Geometry check sheet. Reference: the model listing, model coordinates, mm. Face numbers are marked on the shaded views. A direction names the side the tool comes from. Coordinates: 2 decimals unless noted, no trailing zeros. Loops run counter-clockwise (first coordinate to the right, second up) from the corner with the lowest first, then second, coordinate; pieces in that order, holes last.
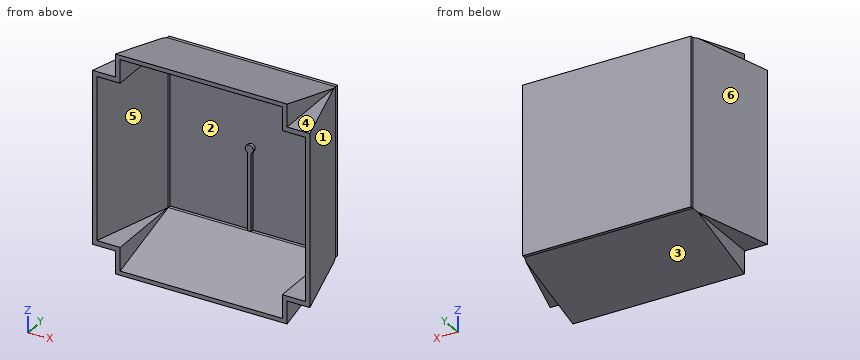
from build123d import *

# Parameters (mm, degrees)
SALIENTE_EXTRUIR1_DEPTH    = 67
CORTAR_EXTRUIR1_DEPTH      = 107
CORTAR_EXTRUIR2_DEPTH      = 107
CORTAR_EXTRUIR3_DEPTH      = 25
CORTAR_EXTRUIR3_DEPTH_BACK = 25
CORTAR_EXTRUIR4_DEPTH      = 25
CORTAR_EXTRUIR4_DEPTH_BACK = 25
CROQUIS14_W                = 7
CROQUIS14_H                = 7
CORTAR_EXTRUIR6_DEPTH      = 70
CROQUIS15_W                = 52
CROQUIS15_H                = 52
SALIENTE_EXTRUIR10_DEPTH   = 1


with BuildPart() as part:
    # Croquis1 → Saliente-Extruir1 (new body)
    with BuildSketch(Plane.XY):
        Polygon((0, 0), (67, 0), (59.5, 26), (7.5, 26), align=None)
    extrude(amount=SALIENTE_EXTRUIR1_DEPTH)

    # Croquis3 → Cortar-Extruir1 (cut)
    with BuildSketch(Plane(origin=(0, 0, 0), x_dir=(0, 0, -1), z_dir=(1, 0, 0))):
        Polygon((-67, 0), (-59.5, 26), (-67, 26), align=None)
        Polygon((0, 0), (-7.5, 26), (0, 26), align=None)
    extrude(amount=CORTAR_EXTRUIR1_DEPTH, mode=Mode.SUBTRACT)

    # Croquis5 → Cortar-Extruir2 (cut)
    with BuildSketch(Plane(origin=(0, 26, 0), x_dir=(1, 0, 0), z_dir=(0, 1, 0))):
        with BuildLine():
            Line((33, -32.354356076), (33, -8.5))
            Line((33, -8.5), (8.5, -8.5))
            Line((8.5, -8.5), (8.5, -58.5))
            Line((8.5, -58.5), (58.5, -58.5))
            Line((58.5, -58.5), (58.5, -8.5))
            Line((58.5, -8.5), (34, -8.5))
            Line((34, -8.5), (34, -32.354356076))
            ThreePointArc((34, -32.354356076), (33.5, -34.75), (33, -32.354356076))
        make_face()
    extrude(amount=-CORTAR_EXTRUIR2_DEPTH, mode=Mode.SUBTRACT)

    # Croquis6 → Cortar-Extruir3 (cut, two sides: drawn at the far end of the back side and taken through both)
    with BuildSketch(Plane(origin=(33.5, 0, 0), x_dir=(0, 0, -1), z_dir=(1, 0, 0)).offset(-CORTAR_EXTRUIR3_DEPTH_BACK)):
        Polygon((-65.711538462, 0), (-58.5, 25), (-8.5, 25), (-1.288461538, 0), align=None)
    extrude(amount=CORTAR_EXTRUIR3_DEPTH + CORTAR_EXTRUIR3_DEPTH_BACK, mode=Mode.SUBTRACT)

    # Croquis7 → Cortar-Extruir4 (cut, two sides: drawn at the far end of the back side and taken through both)
    with BuildSketch(Plane.XY.offset(33.5).offset(-CORTAR_EXTRUIR4_DEPTH_BACK)):
        Polygon((1.288461538, 0), (8.5, 25), (58.5, 25), (65.711538462, 0), align=None)
    extrude(amount=CORTAR_EXTRUIR4_DEPTH + CORTAR_EXTRUIR4_DEPTH_BACK, mode=Mode.SUBTRACT)

    # Croquis14 → Cortar-Extruir6 (cut)
    with BuildSketch(Plane.XZ):
        with Locations((63.5, 3.5)):
            Rectangle(CROQUIS14_W, CROQUIS14_H)
        with Locations((63.5, 63.5)):
            Rectangle(CROQUIS14_W, CROQUIS14_H)
        with Locations((3.5, 3.5)):
            Rectangle(CROQUIS14_W, CROQUIS14_H)
        with Locations((3.5, 63.5)):
            Rectangle(CROQUIS14_W, CROQUIS14_H)
    extrude(amount=-CORTAR_EXTRUIR6_DEPTH, mode=Mode.SUBTRACT)

    # Croquis15 → Saliente-Extruir10 (add)
    with BuildSketch(Plane(origin=(0, 26, 0), x_dir=(1, 0, 0), z_dir=(0, 1, 0))):
        with Locations((33.5, -33.5)):
            Rectangle(CROQUIS15_W, CROQUIS15_H)
    extrude(amount=SALIENTE_EXTRUIR10_DEPTH)


solid = part.part
(1) Access from +Z, -Z, +X, -X, +Y, -Y to the whole of each face (thin tool, end or side, straight path). Record for the marked faces 5 and 6.
Findings:
face 5: -Y
face 6: +Z, -Z, -X, +Y
(2) Draft check along Z on the marked faces 1, 2, 3 and 4. Enter one of: +Z half, -Z half, draft (parallel to the pull), parting line (faces both ways), or undercut.
Findings:
face 1: draft
face 2: undercut
face 3: -Z half
face 4: +Z half
(3) Sectioned sample at B-B on y = 18.25. Record the cut outline in (x, z), and give its area (3 significant figures).
Findings:
outline: (5.26, 7) - (7, 7) - (7, 5.26) - (60, 5.26) - (60, 7) - (61.74, 7) - (61.74, 60) - (60, 60) - (60, 61.74) - (7, 61.74) - (7, 60) - (5.26, 60) - close; hole (6.55, 8.5) - (8.5, 8.5) - (8.5, 6.55) - (58.5, 6.55) - (58.5, 8.5) - (60.45, 8.5) - (60.45, 58.5) - (58.5, 58.5) - (58.5, 60.45) - (8.5, 60.45) - (8.5, 58.5) - (6.55, 58.5) - close
area: 288 mm2
(4) Scan lines: L1, parallel to X at y = 18, z = 31; L2, parallel to Z at x = 54.5, y = 18.75; L3, parallel to Z at x = 54.5, y = 1.5. Record each from-to range of solid material in increasing order.
Findings:
L1: x = 5.19 to 6.48, 60.52 to 61.81
L2: z = 5.41 to 6.7, 60.3 to 61.59
L3: z = 0.43 to 1.72, 65.28 to 66.57
(5) Sectioned sample at A-A on z = 25. Record the cut outline in (x, y).
Findings:
outline: (0, 0) - (1.29, 0) - (8.5, 25) - (8.5, 26) - (33, 26) - (33, 25) - (34, 25) - (34, 26) - (58.5, 26) - (58.5, 25) - (65.71, 0) - (67, 0) - (59.5, 26) - (59.5, 27) - (7.5, 27) - (7.5, 26) - close
(6) Gauge pin test, flat ends, axial feed: pin 1 Ø5 at (y, z) = (12, 16.5) entering from -X; pin 2 Ø3.5 at (y, z) = (11, 62.5) entering from -X; pin 3 Ø1.5 at (y, z) = (19.5, 41) entering from +X. Record the tip position at first contact, or that the pin passes through.
Findings:
pin 1: stops at x = 2.74
pin 2: stops at x = 7
pin 3: stops at x = 61.59
(7) Sectioned sample at C-C on x = 21. Record the cut outline in (y, z).
Findings:
outline: (0, 0) - (26, 7.5) - (27, 7.5) - (27, 59.5) - (26, 59.5) - (0, 67) - (0, 65.71) - (25, 58.5) - (26, 58.5) - (26, 8.5) - (25, 8.5) - (0, 1.29) - close
(8) Sectioned sample at D-D on z = 33.5. Record the cut outline in (x, y), and give its area (3 significant figures).
Findings:
outline: (0, 0) - (1.29, 0) - (8.5, 25) - (8.5, 26) - (32.25, 26) - (32.25, 25) - (34.75, 25) - (34.75, 26) - (58.5, 26) - (58.5, 25) - (65.71, 0) - (67, 0) - (59.5, 26) - (59.5, 27) - (7.5, 27) - (7.5, 26) - close
area: 121 mm2
